Autodesk Inventor part; units mm, degrees
ref_plane "YZ Plane" through (0, 0, 0) normal (1, 0, 0) x (0, 1, 0)
ref_plane "XZ Plane" through (0, 0, 0) normal (0, 1, 0) x (-1, 0, 0)
ref_plane "XY Plane" through (0, 0, 0) normal (0, 0, 1) x (1, 0, 0)
sketch "Sketch1" plane through (0, 0, 0) normal (0, 1, 0) x (-1, 0, 0)
  circle A0 centre (0, 0) radius 2.78
  circle A1 centre (0, 0) radius 2.045
  dimension "d0" = 5.56
  dimension "d1" = 4.09
extrude "Extrusion1" add sketch "Sketch1" along normal blind 8
sketch "Sketch2" plane through (0, 0, 0) normal (0, -1, 0) x (1, 0, 0)
  circle A0 centre (0, 0) radius 1.905
  dimension "d4" = 3.81
extrude "Extrusion2" add sketch "Sketch2" along normal blind 1.524
sketch "Sketch3" plane through (0, 0, 0) normal (0, -1, 0) x (1, 0, 0)
  circle A0 centre (0, 0) radius 2.78
extrude "Extrusion3" add sketch "Sketch3" against normal up to surface (8 mm away)
sketch "Sketch4" plane through (0, 8, 0) normal (0, 1, 0) x (1, 0, 0)
  point P0 (0, 0)
  point P1 (0, 0)
hole "Hole1" at (0, 8, 0) direction (0, -1, 0) diameter 2.4638 end through all
properties part number "Keystone24884" material "Aluminum 6061"
Design review of the part built by this model. Coordinates are the model's own, in mm. A direction names the side the tool comes from. Coordinates: 2 decimals unless noted, no trailing zeros. Order: outer loops, then holes, each group sorted by start corner. A loop starts at its lowest first (then second) coordinate and runs counter-clockwise, first axis right, second up. Notation, with made-up numbers: M -40,35.25 L -22,35.25 A4 cw -22,40.25 Z; hole C 70,15.5 d1. An arc over 180 degrees is marked long. Answer as a JSON object with one key per item and string values. Group by question number.
1) Mouldability with a two-part tool opening along X and no side actions: class faces 3 (the flat face through (-1, -1.524, 1)), 4 (the cylindrical face through (2.2, 3.9, 1.7)), 5 (the cylindrical face through (-0.05, 3.17, -1.23)) as pulls with the +X half, pulls with the -X half, needs draft (parallel to the pull), parting line crosses it, or undercut.
2) Add section D-D, the plane y = 4.5. Write out the cut boundary in (x, z).
3) For pin 1 (1 mm diameter, centred on y = 5.5, z = 1.5, fed in from +X), flat-tipped, find the tip position at first contact; note if it passes through.
4) Wall thickness on L1, parallel to Z at x = 0, y = 3.5; L2, parallel to Y at x = 0.5, z = 2.4: over which ranges is each line inside the solid? List them lowest first.
5) Add section B-B, the plane x = 0. Write out the cut boundary in (y, z) (3 decimals).
6) Tool access review of faces 1 (the flat face through (1, 0, -2)), 2 (the flat face through (-1, 8, -1)): name each direction out of +Z, -Z, +X, -X, +Y, -Y from which nothing blocks a thin tool from reaching the whole face with its end or side.
7) Add section A-A, the plane z = 0. Write out the cut boundary in (x, y) (3 decimals).
8) Add section C-C, the plane y = -1. Write out the cut boundary in (x, z) (3 decimals).
Computed values:
{
 "1": {"face 3": "needs draft", "face 4": "parting line crosses it", "face 5": "undercut"},
 "2": {"outline": "C 0,0 d5.56; hole C 0,0 d2.46"},
 "3": {"pin 1": "stops at x = 2.59"},
 "4": {"L1": "z = -2.78 to -1.23, 1.23 to 2.78", "L2": "y = 0 to 8"},
 "5": {"outline": "M -1.524,-1.905 L 0,-1.905 L 0,-2.78 L 8,-2.78 L 8,-1.232 L -1.524,-1.232 Z; M -1.524,1.232 L 8,1.232 L 8,2.78 L 0,2.78 L 0,1.905 L -1.524,1.905 Z"},
 "6": {"face 1": "-Y", "face 2": "+Z, -Z, +X, -X, +Y"},
 "7": {"outline": "M -2.78,0 L -1.905,0 L -1.905,-1.524 L -1.232,-1.524 L -1.232,8 L -2.78,8 Z; M 1.232,-1.524 L 1.905,-1.524 L 1.905,0 L 2.78,0 L 2.78,8 L 1.232,8 Z"},
 "8": {"outline": "C 0,0 d3.81; hole C 0,0 d2.464"}
}
